```python
from build123d import *

# Parameters (mm, degrees)
F0_R     = 2
F0_R_2   = 1.5
F1_DEPTH = 3
F2_R     = 1


# Not quite as in the source:
# - a fillet or chamfer that OpenCascade refuses, or shapes differently, is made with other operations: its cross-section is extruded or revolved along the edge and cut away or added


with BuildPart() as f1:
    # F0 (on Front) → F1 (new body)
    with BuildSketch(Plane.XZ):
        with BuildLine():
            Line((59.5, 15.5), (-59.5, 15.5))
            ThreePointArc((-59.5, 15.5), (-75, 0), (-59.5, -15.5))
            Line((-59.5, -15.5), (59.5, -15.5))
            ThreePointArc((59.5, -15.5), (75, 0), (59.5, 15.5))
        make_face()
        with Locations((-69.59, 0)):
            Circle(F0_R, mode=Mode.SUBTRACT)
        with Locations((-48, 0)):
            Circle(F0_R_2, mode=Mode.SUBTRACT)
        with Locations((48, 0)):
            Circle(F0_R_2, mode=Mode.SUBTRACT)
        with Locations((71, 0)):
            Circle(F0_R, mode=Mode.SUBTRACT)
    extrude(amount=F1_DEPTH)

    # F2
    f2_edges = [f1.edges().sort_by_distance(p)[0] for p in [
        (0, -3, 15.5),
        (-75, -3, 0),
        (0, -3, -15.5),
        (75, -3, 0),
    ]]
    fillet(f2_edges, radius=F2_R)

    # F3: chamfer of 1.5 on 2 edges, made by hand

    # F3_s1 → F3_t2 (revolve, cut)
    with BuildSketch(Plane.XY):
        Polygon((-66.09, -3), (-67.59, -1.5), (-67.59, -3), align=None)
    revolve(axis=Axis((-69.59, -3, 0), (0, -1, 0)), mode=Mode.SUBTRACT)

    # F3_s3 → F3_t4 (revolve, cut)
    with BuildSketch(Plane.XY):
        Polygon((74.5, -3), (73, -1.5), (73, -3), align=None)
    revolve(axis=Axis((71, -3, 0), (0, -1, 0)), mode=Mode.SUBTRACT)


solid = f1.part
```
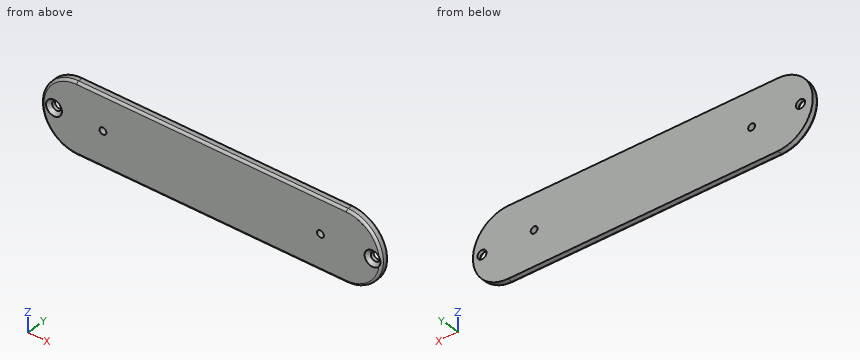
Part model, mm, in its own coordinate system. Coordinates: 2 decimals unless noted, no trailing zeros. Write each loop counter-clockwise with the first axis right and the second up, starting at its lowest first coordinate (ties: lowest second). Pieces come first, ordered by that corner, then holes.
Item 1: Slice it at A-A (x = 48). Write the cut outline in (y, z), and give its area (3 significant figures).
Item 2: Probe line 1 (Z direction, x = 48, y = -2.1); line 2 (X direction, y = -2.2, z = 2); line 3 (X direction, y = -2.05, z = 1). List the from-to ranges inside material, lowest first.
Item 3: Pin check, flat tip, straight feed: pin 1 (6.5 mm diameter, centred on x = 71, z = 0, fed in from -Y). Stop position of the tip, or through.
Item 4: Slice it at B-B (y = -0.8). Write the cut outline in (x, z), and give its area (3 significant figures).
Results found:
1. outline: (-3, -14.5) arc R1 ccw to (-2, -15.5) - (0, -15.5) - (0, -1.5) - (-3, -1.5) - close; (-3, 1.5) - (0, 1.5) - (0, 15.5) - (-2, 15.5) arc R1 ccw to (-3, 14.5) - close
1. area: 83.6 mm2
2. line 1: z = -15.49 to -1.5, 1.5 to 15.49
2. line 2: x = -74.85 to -71.4, -67.78 to 69.19, 72.81 to 74.85
2. line 3: x = -74.97 to -71.94, -67.24 to -49.12, -46.88 to 46.88, 49.12 to 68.65, 73.35 to 74.97
3. pin 1: stops at y = -2.75
4. outline: (-59.5, -15.5) - (59.5, -15.5) arc R15.5 ccw to (59.5, 15.5) - (-59.5, 15.5) arc R15.5 ccw to start; hole circle Ø4 at (-69.59, 0); hole circle Ø3 at (-48, 0); hole circle Ø3 at (48, 0); hole circle Ø4 at (71, 0)
4. area: 4,400 mm2
